```python
from build123d import *

# Parameters (mm, degrees)
F1_DEPTH = 30
F3_DEPTH = 70


with BuildPart() as f1:
    # F0 (on Front) → F1 (new body)
    with BuildSketch(Plane.XZ):
        with BuildLine():
            Line((-27, 0), (0, 0))
            Line((0, 0), (27, 0))
            Line((27, 0), (34.214952, 20.442363))
            ThreePointArc((34.214952, 20.442363), (34.428223, 21.262295), (34.5, 22.106464))
            Line((34.5, 22.106464), (34.5, 42.5))
            Line((34.5, 42.5), (32.5, 42.5))
            Line((32.5, 42.5), (32.5, 21.592585))
            Line((32.5, 21.592585), (25.58497, 2))
            Line((25.58497, 2), (0, 2))
            Line((0, 2), (-25.58497, 2))
            Line((-25.58497, 2), (-32.5, 21.592585))
            Line((-32.5, 21.592585), (-32.5, 42.5))
            Line((-32.5, 42.5), (-34.5, 42.5))
            Line((-34.5, 42.5), (-34.5, 22.106464))
            ThreePointArc((-34.5, 22.106464), (-34.428223, 21.262295), (-34.214952, 20.442363))
            Line((-34.214952, 20.442363), (-27, 0))
        make_face()
    extrude(amount=F1_DEPTH)

    # F2 (on face) → F3 (cut)
    with BuildSketch(Plane(origin=(-34.5, 0, 0), x_dir=(0, -1, 0), z_dir=(-1, 0, 0))):
        with BuildLine():
            ThreePointArc((2.5, 37.5), (2.323223, 37.426777), (2.25, 37.25))
            Line((2.25, 37.25), (2.25, 28))
            ThreePointArc((2.25, 28), (2.542893, 27.292893), (3.25, 27))
            Line((3.25, 27), (26.75, 27))
            ThreePointArc((26.75, 27), (27.457107, 27.292893), (27.75, 28))
            Line((27.75, 28), (27.75, 37.25))
            ThreePointArc((27.75, 37.25), (27.676777, 37.426777), (27.5, 37.5))
            Line((27.5, 37.5), (2.5, 37.5))
        make_face()
    extrude(amount=-F3_DEPTH, mode=Mode.SUBTRACT)


solid = f1.part
```
The model under review builds one solid part; all positions refer to its coordinate system, in mm. A direction names the side the tool comes from. Round coordinates to 2 decimals unless told otherwise and drop trailing zeros. Loops run counter-clockwise (first coordinate to the right, second up) from the corner with the lowest first, then second, coordinate; pieces in that order, holes last. Notation, with made-up numbers: M 8.5,11.5 L 23.5,11.5 A18 cw 23.5,38.5 Z; hole C 68,-37 d4. An arc over 180 degrees is marked long. Write item = value, one per line.
Item 1: The part is to be moulded in two halves that separate along Z. For faces 1 (the flat face through (33, -15, 27)), 2 (the flat face through (33, -15, 37.5)), 3 (the flat face through (0, 0, 1)), 4 (the flat face through (30.557, -14.79, 10.078)), say which applies: released by +Z, released by -Z, zero draft, split by the parting line, or undercut.
Return value:
face_1 = undercut
face_2 = undercut
face_3 = zero draft
face_4 = released by -Z
Item 2: Take a section at B-B on z = 34.5. Write out the cut boundary in (x, y).
Return value:
outline = M -34.5,-30 L -32.5,-30 L -32.5,-27.75 L -34.5,-27.75 Z; M -34.5,-2.25 L -32.5,-2.25 L -32.5,0 L -34.5,0 Z; M 32.5,-30 L 34.5,-30 L 34.5,-27.75 L 32.5,-27.75 Z; M 32.5,-2.25 L 34.5,-2.25 L 34.5,0 L 32.5,0 Z
Item 3: Take a section at A-A on y = -17. Write out the cut boundary in (x, z).
Return value:
outline = M -34.5,22.11 A5 ccw -34.21,20.44 L -27,0 L 27,0 L 34.21,20.44 A5 ccw 34.5,22.11 L 34.5,27 L 32.5,27 L 32.5,21.59 L 25.58,2 L -25.58,2 L -32.5,21.59 L -32.5,27 L -34.5,27 Z; M -34.5,37.5 L -32.5,37.5 L -32.5,42.5 L -34.5,42.5 Z; M 32.5,37.5 L 34.5,37.5 L 34.5,42.5 L 32.5,42.5 Z
Item 4: Insertion check: P1, Ø2, axis at x = -22.5, y = -23, coming from the +Z side; P2, Ø1.5, axis at y = -3.5, z = 21, coming from the +X side. Each pin has a flat end and moves straight along its axis. Give the tip position at first contact, or say it passes through.
Return value:
P1 = 2
P2 = 34.49
Item 5: Take a section at D-D on x = -23. Write out the cut boundary in (y, z).
Return value:
outline = M -30,0 L 0,0 L 0,2 L -30,2 Z
Item 6: For line 1 (X direction, y = -18, z = 39); line 2 (Z direction, x = 23.5, y = -5.5); line 3 (X direction, y = -2.75, z = 6), list the stretches that pass through material, from the lowest coordinate up. Write a range as [from, to].
Return value:
line_1 = [-34.5, -32.5], [32.5, 34.5]
line_2 = [0, 2]
line_3 = [-29.12, -27], [27, 29.12]
Item 7: Take a section at C-C on z = 15.5. Write out the cut boundary in (x, y), then the cut area to 3 significant figures.
Return value:
outline = M -32.47,-30 L -30.35,-30 L -30.35,0 L -32.47,0 Z; M 30.35,-30 L 32.47,-30 L 32.47,0 L 30.35,0 Z
area = 127 mm2
Item 8: Machinability: for faces 5 (the flat face through (-33, -15, 42.5)), 6 (the flat face through (0, -15, 2)), 7 (the flat face through (-34, -27.75, 33)), which of the approach directions +Z, -Z, +X, -X, +Y, -Y give a long, thin tool a straight path to every point of the face, cutting with its end or side? Answer none if there is none.
Return value:
face_5 = +Z, +X, -X, +Y, -Y
face_6 = +Z, +Y, -Y
face_7 = +X, -X
